from build123d import *

# Parameters (mm, degrees)
SKETCH1_W                                       = 38.1
SKETCH1_H                                       = 23.876
GEARBOX_MOUNT_DEPTH                             = 48.26
CBORE_FOR_4_SOCKET_HEAD_CAP_SCREW1_D            = 3.2639
CBORE_FOR_4_SOCKET_HEAD_CAP_SCREW1_DEPTH        = 12.7
CBORE_FOR_4_SOCKET_HEAD_CAP_SCREW1_CBORE_D      = 3.96875
CBORE_FOR_4_SOCKET_HEAD_CAP_SCREW1_CBORE_DEPTH  = 4.7625
CBORE_FOR_4_SOCKET_HEAD_CAP_SCREW1_TIP          = 0.980574487
INSERT_INSTALLATION_CHAMFERS_SIZE               = 0.508
SKETCH7_W                                       = 38.1
SKETCH7_H                                       = 23.876
MOTOR_MOUNT_EXTENSION_DEPTH                     = 41.5798
CBORE_FOR_10_SOCKET_HEAD_CAP_SCREW1_D           = 5.1054
CBORE_FOR_10_SOCKET_HEAD_CAP_SCREW1_CBORE_D     = 9.525
CBORE_FOR_10_SOCKET_HEAD_CAP_SCREW1_CBORE_DEPTH = 4.826
MOTOR_MOUNT_PLATE_DEPTH                         = 6.35
SHAFT_CLEARANCE_REACH                           = 111.391
SKETCH9_R                                       = 4.7625
CSK_FOR_M3_FLAT_HEAD_MACHINE_SCREW1_AT_2_COUNT  = 2
CSK_FOR_M3_FLAT_HEAD_MACHINE_SCREW1_AT_2_PITCH  = 19
CSK_FOR_M3_FLAT_HEAD_MACHINE_SCREW1_AT_3_COUNT  = 2
CSK_FOR_M3_FLAT_HEAD_MACHINE_SCREW1_AT_3_PITCH  = 15.700318468
CSK_FOR_M3_FLAT_HEAD_MACHINE_SCREW1_AT_4_COUNT  = 2
CSK_FOR_M3_FLAT_HEAD_MACHINE_SCREW1_AT_4_PITCH  = 15.700318468
CHAMFER2_SIZE                                   = 12.7
CUT_EXTRUDE1_REACH                              = 78.048
SKETCH12_R                                      = 2.6035
SKETCH13_R                                      = 1.73482
CUT_EXTRUDE2_DEPTH                              = 104.851713072


with BuildPart() as part:
    # Sketch1 → Gearbox Mount (new body)
    with BuildSketch(Plane.XY):
        Rectangle(SKETCH1_W, SKETCH1_H)
    extrude(amount=GEARBOX_MOUNT_DEPTH)

    # CBORE for #4 Socket Head Cap Screw1
    with Locations(Plane(origin=(0, 11.938, 0), x_dir=(1, 0, 0), z_dir=(0, 1, 0))):
        with Locations((0, -3.81), (-9.525, -22.225), (0, -40.64), (9.525, -22.225)):
            CounterBoreHole(CBORE_FOR_4_SOCKET_HEAD_CAP_SCREW1_D / 2, CBORE_FOR_4_SOCKET_HEAD_CAP_SCREW1_CBORE_D / 2, CBORE_FOR_4_SOCKET_HEAD_CAP_SCREW1_CBORE_DEPTH, depth=CBORE_FOR_4_SOCKET_HEAD_CAP_SCREW1_DEPTH)
            with Locations((0, 0, -(CBORE_FOR_4_SOCKET_HEAD_CAP_SCREW1_DEPTH + CBORE_FOR_4_SOCKET_HEAD_CAP_SCREW1_TIP / 2))):  # 118° drill point
                Cone(0, CBORE_FOR_4_SOCKET_HEAD_CAP_SCREW1_D / 2, CBORE_FOR_4_SOCKET_HEAD_CAP_SCREW1_TIP, mode=Mode.SUBTRACT)

    # Insert Installation Chamfers
    insert_installation_chamfers_edges = [part.edges().sort_by_distance(p)[0] for p in [
        (7.540625, 11.938, 22.225),
        (-1.984375, 11.938, 40.64),
        (-11.509375, 11.938, 22.225),
        (-1.984375, 11.938, 3.81),
    ]]
    chamfer(insert_installation_chamfers_edges, length=INSERT_INSTALLATION_CHAMFERS_SIZE)

    # Sketch7 → Motor Mount Extension (add)
    with BuildSketch(Plane(origin=(0, 0, 0), x_dir=(-1, 0, 0), z_dir=(0, 0, -1))):
        Rectangle(SKETCH7_W, SKETCH7_H)
    extrude(amount=MOTOR_MOUNT_EXTENSION_DEPTH)

    # CBORE for #10 Socket Head Cap Screw1 (through all)
    with Locations(Plane(origin=(0, 11.938, 0), x_dir=(1, 0, 0), z_dir=(0, 1, 0))):
        with Locations((-9.525, -40.64), (9.525, -40.64), (9.525, -3.81), (-9.525, -3.81)):
            CounterBoreHole(CBORE_FOR_10_SOCKET_HEAD_CAP_SCREW1_D / 2, CBORE_FOR_10_SOCKET_HEAD_CAP_SCREW1_CBORE_D / 2, CBORE_FOR_10_SOCKET_HEAD_CAP_SCREW1_CBORE_DEPTH)

    # Sketch8 → Motor Mount Plate (add)
    with BuildSketch(Plane(origin=(0, 0, -41.5798), x_dir=(-1, 0, 0), z_dir=(0, 0, -1))):
        with BuildLine():
            Line((19.05, 11.938), (-19.05, 11.938))
            Line((-19.05, 11.938), (-19.05, -11.938))
            Line((-19.05, -11.938), (-17.446279027, -32.358163541))
            ThreePointArc((-17.446279027, -32.358163541), (0, -48.488), (17.446279027, -32.358163541))
            Line((17.446279027, -32.358163541), (19.05, -11.938))
            Line((19.05, -11.938), (19.05, 11.938))
        make_face()
    extrude(amount=MOTOR_MOUNT_PLATE_DEPTH)

    # Sketch9 → Shaft Clearance (cut, up to next)
    with BuildSketch(Plane(origin=(0, 0, -47.9298), x_dir=(-1, 0, 0), z_dir=(0, 0, -1)), mode=Mode.PRIVATE) as shaft_clearance_sk1:
        with Locations((0, -30.988)):
            Circle(SKETCH9_R)
    shaft_clearance_tool1 = extrude(shaft_clearance_sk1.sketch, amount=-SHAFT_CLEARANCE_REACH, mode=Mode.PRIVATE) & part.part
    add(shaft_clearance_tool1.solids().sort_by_distance((0, -30.988, -47.9298))[0], mode=Mode.SUBTRACT)

    # Sketch10 → CSK for M3 Flat Head Machine Screw1 (revolve, cut)
    with BuildSketch(Plane(origin=(9.5, -30.988, -47.9298), x_dir=(0, 1, 0), z_dir=(1, 0, 0))):
        Polygon((0, 0), (0, 6.35), (1.7, 6.35), (1.7, 5.26), (3.15, 3.81), (3.15, 0), align=None)
    csk_for_m3_flat_head_machine_screw1 = revolve(axis=Axis((9.5, -30.988, -54.2798), (0, 0, 1)), mode=Mode.SUBTRACT)

    # CSK for M3 Flat Head Machine Screw1 at 2: CSK for M3 Flat Head Machine Screw1 ×2
    with Locations(*[(-i * CSK_FOR_M3_FLAT_HEAD_MACHINE_SCREW1_AT_2_PITCH, 0, 0) for i in range(1, CSK_FOR_M3_FLAT_HEAD_MACHINE_SCREW1_AT_2_COUNT)]):
        add(csk_for_m3_flat_head_machine_screw1, mode=Mode.SUBTRACT)

    # CSK for M3 Flat Head Machine Screw1 at 3: CSK for M3 Flat Head Machine Screw1 ×2
    with Locations(*[Vector(-0.6050832675335578, 0.7961621941231026, 0) * (i * CSK_FOR_M3_FLAT_HEAD_MACHINE_SCREW1_AT_3_PITCH) for i in range(1, CSK_FOR_M3_FLAT_HEAD_MACHINE_SCREW1_AT_3_COUNT)]):
        add(csk_for_m3_flat_head_machine_screw1, mode=Mode.SUBTRACT)

    # CSK for M3 Flat Head Machine Screw1 at 4: CSK for M3 Flat Head Machine Screw1 ×2
    with Locations(*[Vector(-0.605083267533558, -0.7961621941231024, 0) * (i * CSK_FOR_M3_FLAT_HEAD_MACHINE_SCREW1_AT_4_PITCH) for i in range(1, CSK_FOR_M3_FLAT_HEAD_MACHINE_SCREW1_AT_4_COUNT)]):
        add(csk_for_m3_flat_head_machine_screw1, mode=Mode.SUBTRACT)

    # Chamfer2
    chamfer2_edges = [part.edges().sort_by_distance(p)[0] for p in [
        (0, 11.938, -47.9298),
    ]]
    chamfer(chamfer2_edges, length=CHAMFER2_SIZE)

    # Sketch12 → Cut-Extrude1 (cut, up to next)
    with BuildSketch(Plane(origin=(0, 7.112, 0), x_dir=(1, 0, 0), z_dir=(0, 1, 0)), mode=Mode.PRIVATE) as cut_extrude1_sk1:
        with Locations(Location((-9.525, -3.81, 0), (0, 0, 270))):
            Circle(SKETCH12_R)
    cut_extrude1_tool1 = extrude(cut_extrude1_sk1.sketch, amount=-CUT_EXTRUDE1_REACH, mode=Mode.PRIVATE) & part.part
    # Sketch12 → Cut-Extrude1 (cut, up to next)
    with BuildSketch(Plane(origin=(0, 7.112, 0), x_dir=(1, 0, 0), z_dir=(0, 1, 0)), mode=Mode.PRIVATE) as cut_extrude1_sk2:
        with Locations(Location((9.525, -3.81, 0), (0, 0, 270))):
            Circle(SKETCH12_R)
    cut_extrude1_tool2 = extrude(cut_extrude1_sk2.sketch, amount=-CUT_EXTRUDE1_REACH, mode=Mode.PRIVATE) & part.part
    # Sketch12 → Cut-Extrude1 (cut, up to next)
    with BuildSketch(Plane(origin=(0, 7.112, 0), x_dir=(1, 0, 0), z_dir=(0, 1, 0)), mode=Mode.PRIVATE) as cut_extrude1_sk3:
        with Locations(Location((-9.525, -40.64, 0), (0, 0, 270))):
            Circle(SKETCH12_R)
    cut_extrude1_tool3 = extrude(cut_extrude1_sk3.sketch, amount=-CUT_EXTRUDE1_REACH, mode=Mode.PRIVATE) & part.part
    # Sketch12 → Cut-Extrude1 (cut, up to next)
    with BuildSketch(Plane(origin=(0, 7.112, 0), x_dir=(1, 0, 0), z_dir=(0, 1, 0)), mode=Mode.PRIVATE) as cut_extrude1_sk4:
        with Locations(Location((9.525, -40.64, 0), (0, 0, 270))):
            Circle(SKETCH12_R)
    cut_extrude1_tool4 = extrude(cut_extrude1_sk4.sketch, amount=-CUT_EXTRUDE1_REACH, mode=Mode.PRIVATE) & part.part
    add(cut_extrude1_tool1.solids().sort_by_distance((-9.525, 7.112, 3.81))[0], mode=Mode.SUBTRACT)
    add(cut_extrude1_tool2.solids().sort_by_distance((9.525, 7.112, 3.81))[0], mode=Mode.SUBTRACT)
    add(cut_extrude1_tool3.solids().sort_by_distance((-9.525, 7.112, 40.64))[0], mode=Mode.SUBTRACT)
    add(cut_extrude1_tool4.solids().sort_by_distance((9.525, 7.112, 40.64))[0], mode=Mode.SUBTRACT)

    # Sketch13 → Cut-Extrude2 (cut, through all)
    with BuildSketch(Plane.XY.offset(-41.5798)):
        with Locations((0, -18.488)):
            Circle(SKETCH13_R)
        with Locations((-9.5, -30.988)):
            Circle(SKETCH13_R)
        with Locations((9.5, -30.988)):
            Circle(SKETCH13_R)
        with Locations((0, -43.488)):
            Circle(SKETCH13_R)
    extrude(amount=-CUT_EXTRUDE2_DEPTH, mode=Mode.SUBTRACT)


solid = part.part
The listing builds one solid part. Answer for the finished solid, in the listing's coordinates (mm). A direction names the side the tool comes from. Coordinates: 2 decimals unless noted, no trailing zeros. Loops run counter-clockwise (first coordinate to the right, second up) from the corner with the lowest first, then second, coordinate; pieces in that order, holes last.
1) Find section A-A on y = 3. Give the number of separate pieces and of enclosed holes in the cut face, then the cut area to 3 significant figures.
2) Flat-ended cylindrical pins translate along their axes: pin 1 Ø5 at (x, z) = (-11.5, 40) entering from +Y; pin 2 Ø10 at (x, y) = (0, -18.488) entering from +Z; pin 3 Ø7.5 at (x, z) = (9.525, 3.81) entering from -Y. Find the tip coordinate at first contact, or state that the pin passes through.
3) A tool of negligible diameter and unlimited length cuts with its end or side. For faces 1 (the face through (0.354, 3.151, 5.403)), 2 (the face through (0.62, -26.266, -44.799)), 3 (the face through (7.37, -33.31, -46.05)), 4 (the face through (0, -11.938, 4)), from which of +Z, -Z, +X, -X, +Y, -Y can it reach the whole face along a straight path? Write none if from no direction.
4) Find the intervals of material crossed by L1, parallel to X at y = 10.7, z = 40.64; L2, parallel to X at y = -7.25, z = 3.81; L3, parallel to Z at x = -8.5, y = 7, in increasing order.
5) Determine the mould class of faces 5 (the face through (19.05, 0, 1)), 6 (the face through (0, -24, -47.93)), 7 (the face through (-0.877, 3.151, 39.264)) for opening direction X: pulls with the +X half, pulls with the -X half, needs draft (parallel to the pull), parting line crosses it, or undercut.
6) Find section B-B on z = -32. Write down the section's boundary in (x, y), then the cut area to 3 significant figures.
Values:
1. separate pieces: 1
1. enclosed holes: 8
1. area: 3,400 mm2
2. pin 1: stops at y = 7.11
2. pin 2: stops at z = -41.58
2. pin 3: stops at y = -11.94
3. face 1: +Y
3. face 2: +Z, -Z
3. face 3: -Z
3. face 4: +Z, +X, -X, -Y
4. L1: x = -19.05 to -14.29, -4.76 to -1.98, 1.98 to 4.76, 14.29 to 19.05
4. L2: x = -19.05 to -12.13, -6.92 to 6.92, 12.13 to 19.05
4. L3: z = -40.17 to 1.42, 6.2 to 20.96, 23.49 to 38.25, 43.03 to 48.26
5. face 5: pulls with the +X half
5. face 6: needs draft
5. face 7: undercut
6. outline: (-19.05, -11.94) - (19.05, -11.94) - (19.05, 11.94) - (-19.05, 11.94) - close
6. area: 910 mm2
